Can you work these out from the model? Positions are in its coordinate system, mm. Face numbers are marked on the shaded views. A direction names the side the tool comes from. Give positions to 0.01 mm unless a question says otherwise; leave off trailing zeros. Order: outer loops, then holes, each group sorted by start corner. A loop starts at its lowest first (then second) coordinate and runs counter-clockwise, first axis right, second up. Notation, with made-up numbers: M 67.5,61 L 84.5,61 A21 cw 84.5,83 Z; hole C 89.5,61.5 d11. An arc over 180 degrees is marked long. One line per question, with ' | ' between items. Start each with the question number.
1) If we section it at C-C, the plane y = 37: Please give me the cut outline in (x, z), plus the area to 3 significant figures.
2) If we section it at A-A, the plane x = 31: Please give me the cut outline in (y, z).
3) I'm going to push flat-ended pins straight in: pin 1 Ø2 at (x, z) = (21.5, 19) entering from +Y; pin 2 Ø6 at (y, z) = (33, -6.5) entering from +X; pin 3 Ø5 at (y, z) = (38.5, -4) entering from +X. Where does each tip first touch, or does it pass through?
4) For the marked faces 1 and 2, which set-ups out of +Z, -Z, +X, -X, +Y, -Y let a thin tool reach every point of the face, with its end or its side?
5) Please list where these lines run through material, in increasing order: line 1 along Z through (x, y) = (26.5, 37.5); line 2 along X through (y, z) = (17.5, -18); line 3 along Y through (x, z) = (23.5, -17.5). Write a range as [from, to].
6) If we section it at D-D, the plane z = 3.5: Please give me the cut outline in (x, y).
7) If we section it at B-B, the plane z = -17.5: Please give me the cut outline in (x, y), plus the area to 3 significant figures.
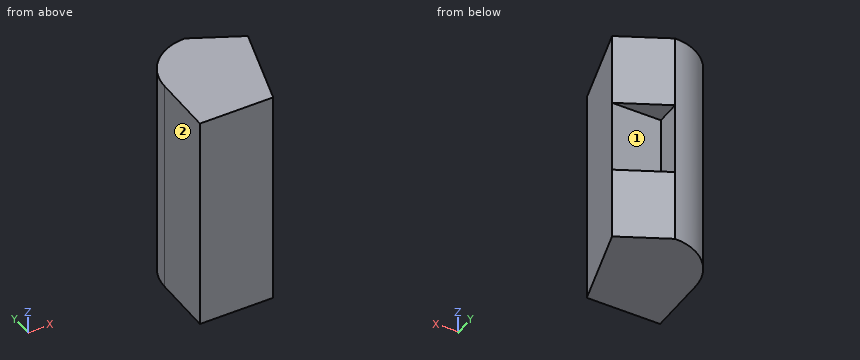
```python
from build123d import *

# Parameters (mm, degrees)
BOSS_EXTRUDE1_DEPTH = 45
CUT_EXTRUDE1_DEPTH  = 15


with BuildPart() as part:
    # Sketch1 → Boss-Extrude1 (new, symmetric)
    with BuildSketch(Plane.XY):
        with BuildLine():
            Line((20, 45), (20, 35))
            Line((20, 35), (40, 35))
            Line((40, 35), (30, 0))
            Line((30, 0), (0, 0))
            Line((0, 0), (0, 25))
            ThreePointArc((0, 25), (5.857864376, 39.142135624), (20, 45))
        make_face()
        Polygon((20, 45), (40, 35), (20, 35), align=None)
    extrude(amount=BOSS_EXTRUDE1_DEPTH, both=True)

    # Sketch1_3 → Cut-Extrude1 (cut, symmetric)
    with BuildSketch(Plane.XY):
        Polygon((20, 45), (40, 35), (20, 35), align=None)
    extrude(amount=CUT_EXTRUDE1_DEPTH, both=True, mode=Mode.SUBTRACT)


solid = part.part
```
Results found:
1) outline: M 4,-45 L 36,-45 L 36,-15 L 20,-15 L 20,15 L 36,15 L 36,45 L 4,45 Z | area: 2,400 mm²
2) outline: M 3.5,-45 L 39.5,-45 L 39.5,-15 L 35,-15 L 35,15 L 39.5,15 L 39.5,45 L 3.5,45 Z
3) pin 1: stops at y = 44.75 | pin 2: stops at x = 40 | pin 3: stops at x = 20
4) face 1: +X, +Y | face 2: +Z, -Z, -X, +Y, -Y
5) line 1: z = [-45, -15], [15, 45] | line 2: x = [0, 35] | line 3: y = [0, 43.25]
6) outline: M 0,0 L 30,0 L 40,35 L 20,35 L 20,45 A20 ccw 0,25 Z
7) outline: M 0,0 L 30,0 L 40,35 L 20,45 A20 ccw 0,25 Z | area: 1,440 mm²
